```python
from build123d import *

# Parameters (mm, degrees)
F2_DEPTH = 12.7
F0_W     = 44.45
F0_H     = 31.75
F3_DEPTH = 12.7
F5_DEPTH = 25.4
F7_DEPTH = 25.4


with BuildPart() as f2:
    # F1 (on face) → F2 (new body)
    with BuildSketch(Plane.XZ):
        Polygon((0, 12.7), (-44.45, 12.7), (-44.037469, 0), (0, 0), align=None)
    extrude(amount=F2_DEPTH)

    # F0 (on Front) → F3 (join)
    with BuildSketch(Plane.XZ):
        with Locations((-22.225, 15.875)):
            Rectangle(F0_W, F0_H)
    extrude(amount=-F3_DEPTH)

    # F4 (on face) → F5 (cut)
    with BuildSketch(Plane.XZ):
        Polygon((0, 31.75), (-19.05, 31.75), (0, 12.7), align=None)
    extrude(amount=-F5_DEPTH, mode=Mode.SUBTRACT)

    # F6 (on face) → F7 (cut)
    with BuildSketch(Plane.XY.offset(12.7)):
        Polygon((0, 0), (-12.7, -12.7), (0, -12.7), align=None)
    extrude(amount=-F7_DEPTH, mode=Mode.SUBTRACT)


solid = f2.part
```
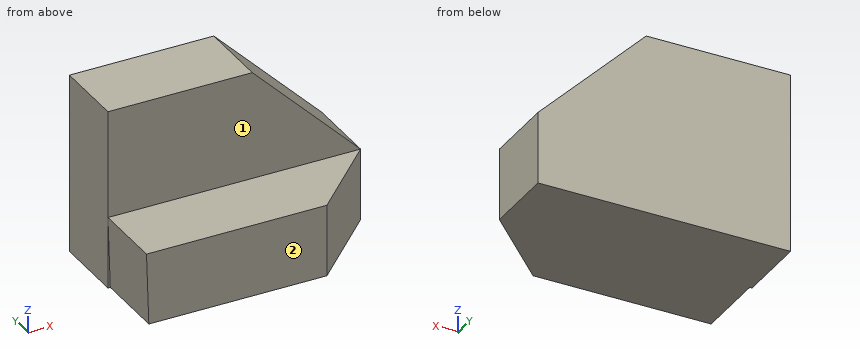
Verification items for the finished model (mm, model axes). Face numbers are marked on the shaded views. A direction names the side the tool comes from. Coordinates: 2 decimals unless noted, no trailing zeros. Write each loop counter-clockwise with the first axis right and the second up, starting at its lowest first coordinate (ties: lowest second). Pieces come first, ordered by that corner, then holes. Notation, with made-up numbers: M 72,-3.75 L 125,-3.75 A9 ccw 125,9.25 Z; hole C -35.75,63.5 d4. An arc over 180 degrees is marked long. Answer as a JSON object with one key per item and string values. Group by question number.
(1) Cross-section at A-A, the plane y = 6.75. Record the cut outline in (x, z).
(2) Cross-section at B-B, the plane x = -4.5. Record the cut outline in (y, z), and give its area (3 significant figures).
(3) Gauge pin test, flat ends, axial feed: pin 1 (3 mm diameter, centred on y = 9.5, z = 24, fed in from +X); pin 2 (12 mm diameter, centred on x = -27, z = 23.5, fed in from -Y); pin 3 (2 mm diameter, centred on y = -1.5, z = 15.5, fed in from +X). Record the tip position at first contact, or that the pin passes through.
(4) Material ranges on line 1 (Y direction, x = -30, z = 14); line 2 (X direction, y = -9.25, z = 5), recorded low to high.
(5) Tool access check on the marked faces 1 and 2. Record the directions out of +Z, -Z, +X, -X, +Y, -Y that give a thin tool (end or side, any length) a straight path to the whole face; none if there is none.
(6) Cross-section at D-D, the plane x = -11. Record the cut outline in (y, z).
Reply:
{
 "1": {"outline": "M -44.45,0 L 0,0 L 0,12.7 L -19.05,31.75 L -44.45,31.75 Z"},
 "2": {"outline": "M -4.5,0 L 12.7,0 L 12.7,17.2 L 0,17.2 L 0,12.7 L -4.5,12.7 Z", "area": "276 mm²"},
 "3": {"pin 1": "x = -9.8", "pin 2": "y = 0", "pin 3": "through"},
 "4": {"line 1": "0 to 12.7", "line 2": "-44.2 to -9.25"},
 "5": {"face 1": "+Z, +X, -X, -Y", "face 2": "+Z, -Z, +X, -X, -Y"},
 "6": {"outline": "M -11,0 L 12.7,0 L 12.7,23.7 L 0,23.7 L 0,12.7 L -11,12.7 Z"}
}
